The listing builds one solid part. Answer for the finished solid, in the listing's coordinates (mm). A direction names the side the tool comes from. Give positions to 0.01 mm unless a question says otherwise; leave off trailing zeros. Order: outer loops, then holes, each group sorted by start corner. A loop starts at its lowest first (then second) coordinate and runs counter-clockwise, first axis right, second up. Notation, with made-up numbers: (22.5, -35.5) - (55.5, -35.5) arc R29 cw to (55.5, -0.5) - close; hole circle Ø8 at (75, 89). An arc over 180 degrees is marked (long way). Answer as a JSON object with one key per item and string values. Group by question number.
Q1. The mould has two halves that part along Y. Classify faces 6 (the face through (8.6, 2, 11.4)), 7 (the face through (25.785, 26.475, -5.772)), 8 (the face through (-23.25, 19, 2)): released by +Y, released by -Y, zero draft, split by the parting line, or undercut.
Q2. A cutting plane is placed at B-B, the plane y = 22. Give the vertices of the cut face in (x, z), and give its area (3 significant figures).
Q3. For faces 1 (the face through (-10.97, 0.99, -8.73)), 2 (the face through (8.6, 2, -8.6)), 3 (the face through (23.25, 19, 3)), 4 (the face through (25.785, 12.21, 6.774)), 5 (the face through (18.25, 19, -17)), determine the directions among +Z, -Z, +X, -X, +Y, -Y from which every point of the face is accessible in a straight line to the end or side of a thin tool.
Q4. Given pin 1 (19.5 mm diameter, centred on x = 6, z = 0.5, fed in from +Y); pin 2 (5 mm diameter, centred on x = 10, z = 10, fed in from +Y); pin 3 (4 mm diameter, centred on x = 20.5, y = 19.5, fed in from +Z), each flat-ended and moving along its own axis, determine where each tip first touches the part or whether it passes through.
Q5. Consider line 1 (X direction, y = 4, z = -10); line 2 (X direction, y = 21.5, z = -7); line 3 (Z direction, x = -24, y = 11). Determine where each line is inside the solid, lowest interval first.
Q6. A cutting plane is placed at C-C, the plane z = 6. Give the vertices of the cut face in (x, y).
Q7. A cutting plane is placed at D-D, the plane y = 11.5. Give the vertices of the cut face in (x, z), and give its area (3 significant figures).
Q8. A cutting plane is placed at A-A, the plane x = -10. Give the vertices of the cut face in (y, z).
from build123d import *

# Parameters (mm, degrees)
SKETCH9_W                                       = 56.5
SKETCH9_H                                       = 39
BOSS_EXTRUDE7_DEPTH                             = 33.5
SKETCH10_R                                      = 1.05
CUT_EXTRUDE2_DEPTH                              = 69.518245745
CUT_EXTRUDE3_DEPTH                              = 28.5
SKETCH12_W                                      = 36.5
SKETCH12_H                                      = 28.5
CUT_EXTRUDE4_DEPTH                              = 56.464515683
CBORE_FOR_M3_SOCKET_HEAD_CAP_SCREW3_D           = 3.2
CBORE_FOR_M3_SOCKET_HEAD_CAP_SCREW3_CBORE_D     = 6.5
CBORE_FOR_M3_SOCKET_HEAD_CAP_SCREW3_CBORE_DEPTH = 3


with BuildPart() as part:
    # Sketch9 → Boss-Extrude7 (new body)
    with BuildSketch(Plane(origin=(0, 0, 0), x_dir=(1, 0, 0), z_dir=(0, 1, 0))):
        Rectangle(SKETCH9_W, SKETCH9_H)
    extrude(amount=BOSS_EXTRUDE7_DEPTH)

    # Sketch10 → Cut-Extrude2 (cut, through all)
    with BuildSketch(Plane(origin=(28.25, 0, 0), x_dir=(0, 0, -1), z_dir=(1, 0, 0))):
        with Locations((-6, 11.5)):
            Circle(SKETCH10_R)
        with Locations(Location((6, 11.5, 0), (0, 0, 180))):
            Circle(SKETCH10_R)
        with Locations((6, 27.5)):
            Circle(SKETCH10_R)
        with Locations(Location((-6, 27.5, 0), (0, 0, 180))):
            Circle(SKETCH10_R)
    extrude(amount=-CUT_EXTRUDE2_DEPTH, mode=Mode.SUBTRACT)

    # Sketch11 → Cut-Extrude3 (cut)
    with BuildSketch(Plane(origin=(0, 33.5, 0), x_dir=(1, 0, 0), z_dir=(0, 1, 0))):
        Polygon((-23.25, -14.5), (-23.25, -19.5), (23.25, -19.5), (23.25, -14.5), (23.25, 14.5), (-23.25, 14.5), align=None)
    extrude(amount=-CUT_EXTRUDE3_DEPTH, mode=Mode.SUBTRACT)

    # Sketch12 → Cut-Extrude4 (cut, through all)
    with BuildSketch(Plane.XY.offset(-14.5)):
        with Locations((0, 19.25)):
            Rectangle(SKETCH12_W, SKETCH12_H)
    extrude(amount=-CUT_EXTRUDE4_DEPTH, mode=Mode.SUBTRACT)

    # CBORE for M3 Socket Head Cap Screw3 (through all)
    with Locations(Plane(origin=(10, 5, -10), x_dir=(0, 0, 1), z_dir=(0, 1, 0))):
        with Locations((0, 0), (20, 0), (20, -20), (0, -20)):
            CounterBoreHole(CBORE_FOR_M3_SOCKET_HEAD_CAP_SCREW3_D / 2, CBORE_FOR_M3_SOCKET_HEAD_CAP_SCREW3_CBORE_D / 2, CBORE_FOR_M3_SOCKET_HEAD_CAP_SCREW3_CBORE_DEPTH)


solid = part.part
Reply:
{
 "1": {"face 6": "released by +Y", "face 7": "undercut", "face 8": "zero draft"},
 "2": {"outline": "(-28.25, -19.5) - (-18.25, -19.5) - (-18.25, -14.5) - (-23.25, -14.5) - (-23.25, 19.5) - (-28.25, 19.5) - close; (18.25, -19.5) - (28.25, -19.5) - (28.25, 19.5) - (23.25, 19.5) - (23.25, -14.5) - (18.25, -14.5) - close", "area": "440 mm^2"},
 "3": {"face 1": "+Y, -Y", "face 2": "+Y", "face 3": "+Z, +Y", "face 4": "+X, -X", "face 5": "+Z, -Z, +Y"},
 "4": {"pin 1": "stops at y = 5", "pin 2": "stops at y = 2", "pin 3": "stops at z = -14.5"},
 "5": {"line 1": "x = -28.25 to -13.25, -6.75 to 6.75, 13.25 to 28.25", "line 2": "x = -28.25 to -23.25, 23.25 to 28.25", "line 3": "z = -19.5 to -6.92, -5.08 to 5.08, 6.92 to 19.5"},
 "6": {"outline": "(-28.25, 0) - (28.25, 0) - (28.25, 10.45) - (23.25, 10.45) - (23.25, 5) - (-23.25, 5) - (-23.25, 10.45) - (-28.25, 10.45) - close; (-28.25, 12.55) - (-23.25, 12.55) - (-23.25, 26.45) - (-28.25, 26.45) - close; (-28.25, 28.55) - (-23.25, 28.55) - (-23.25, 33.5) - (-28.25, 33.5) - close; (23.25, 12.55) - (28.25, 12.55) - (28.25, 26.45) - (23.25, 26.45) - close; (23.25, 28.55) - (28.25, 28.55) - (28.25, 33.5) - (23.25, 33.5) - close"},
 "7": {"outline": "(-28.25, -19.5) - (-18.25, -19.5) - (-18.25, -14.5) - (-23.25, -14.5) - (-23.25, -7.05) - (-28.25, -7.05) - close; (-28.25, -4.95) - (-23.25, -4.95) - (-23.25, 4.95) - (-28.25, 4.95) - close; (-28.25, 7.05) - (-23.25, 7.05) - (-23.25, 19.5) - (-28.25, 19.5) - close; (18.25, -19.5) - (28.25, -19.5) - (28.25, -7.05) - (23.25, -7.05) - (23.25, -14.5) - (18.25, -14.5) - close; (23.25, -4.95) - (28.25, -4.95) - (28.25, 4.95) - (23.25, 4.95) - close; (23.25, 7.05) - (28.25, 7.05) - (28.25, 19.5) - (23.25, 19.5) - close", "area": "398 mm^2"},
 "8": {"outline": "(0, -19.5) - (5, -19.5) - (5, -13.25) - (2, -13.25) - (2, -11.6) - (0, -11.6) - close; (0, -8.4) - (2, -8.4) - (2, -6.75) - (5, -6.75) - (5, 6.75) - (2, 6.75) - (2, 8.4) - (0, 8.4) - close; (0, 11.6) - (2, 11.6) - (2, 13.25) - (5, 13.25) - (5, 19.5) - (0, 19.5) - close"}
}
